Verification items for this drawing (mm, ordinates from the low corner). Give positions to 0.01 mm unless a question says otherwise; leave off trailing zeros. Loops run counter-clockwise (first coordinate to the right, second up) from the corner with the lowest first, then second, coordinate; pieces in that order, holes last. Notation, with made-up numbers: (30, 12.25) -> (80, 12.25) arc R27 cw to (80, 46.25) -> close; hole circle Ø9 at (76, 82.5). An arc over 180 degrees is marked (long way). Answer in a Markdown table with one row per item. Add a question column.
Q1. Material ranges on probe 1 along X at (y, z) = (4.9, 0.3); probe 2 along Y at (x, z) = (95.1, 0.8); probe 3 along Y at (x, z) = (115.1, 1.3), recorded low to high.
Q2. Section check B-B on z = 3.1. Give the number of separate pieces and of enclosed holes in the cut face, and give its area (3 significant figures).
Q3. Section check D-D on x = 114.5. Enter the section's corners in (y, z).
Q4. Section check C-C on x = 85.1. Enter the section's corners in (y, z), and give its area (3 significant figures).
Q5. Gauge pin test, flat ends, axial feed: P1, Ø3, axis at x = 45, y = 44.5, coming from the +Z side; P2, Ø2.5, axis at x = 45.1, y = 4.9, coming from the +Z side. Record the tip position at first contact, or that the pin passes through.
Q6. Section check A-A on y = 24.9. Enter the section's corners in (x, z), and give its area (4 significant figures).
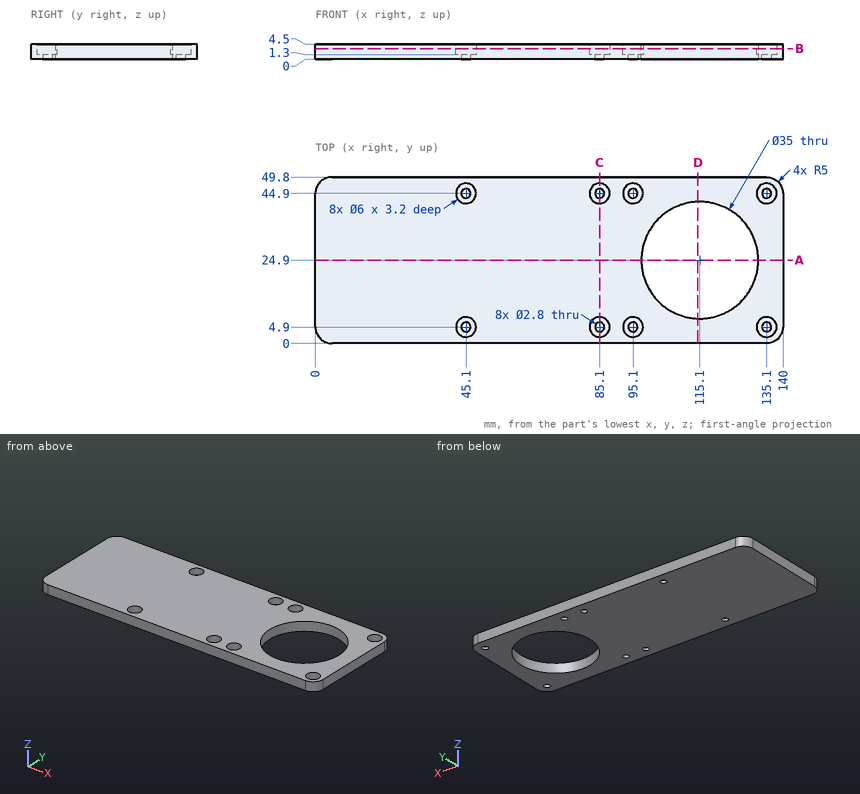
Taken from the geometry:
| question | item | result |
|---|---|---|
| 1 | probe 1 | x = 0 to 43.7, 46.5 to 83.7, 86.5 to 93.7, 96.5 to 133.7, 136.5 to 140 |
| 1 | probe 2 | y = 0 to 3.5, 6.3 to 43.5, 46.3 to 49.8 |
| 1 | probe 3 | y = 0 to 7.4, 42.4 to 49.8 |
| 2 | separate pieces | 1 |
| 2 | enclosed holes | 9 |
| 2 | area | 5,760 mm² |
| 3 | outline | (0, 0) -> (7.41, 0) -> (7.41, 4.5) -> (0, 4.5) -> close; (42.39, 0) -> (49.8, 0) -> (49.8, 4.5) -> (42.39, 4.5) -> close |
| 4 | outline | (0, 0) -> (3.5, 0) -> (3.5, 1.3) -> (1.9, 1.3) -> (1.9, 4.5) -> (0, 4.5) -> close; (6.3, 0) -> (43.5, 0) -> (43.5, 1.3) -> (41.9, 1.3) -> (41.9, 4.5) -> (7.9, 4.5) -> (7.9, 1.3) -> (6.3, 1.3) -> close; (46.3, 0) -> (49.8, 0) -> (49.8, 4.5) -> (47.9, 4.5) -> (47.9, 1.3) -> (46.3, 1.3) -> close |
| 4 | area | 178 mm² |
| 5 | P1 | stops at z = 1.3 |
| 5 | P2 | passes through |
| 6 | outline | (0, 0) -> (97.6, 0) -> (97.6, 4.5) -> (0, 4.5) -> close; (132.6, 0) -> (140, 0) -> (140, 4.5) -> (132.6, 4.5) -> close |
| 6 | area | 472.5 mm² |
